CAD build for the part. Positions are in the model's coordinates, mm. Give positions to 0.01 mm unless a question says otherwise; leave off trailing zeros. Loops run counter-clockwise (first coordinate to the right, second up) from the corner with the lowest first, then second, coordinate; pieces in that order, holes last.
```python
from build123d import *

# Parameters (mm, degrees)
F_01_GASKET_DEPTH  = 1
SKETCH_2_R         = 24
F_02_HOLE_UP_DEPTH = 3
SKETCH_3_R         = 24
F_03_HOLE_LO_DEPTH = 3
SKETCH_4_R         = 4
F_04_BOLT_0_DEPTH  = 3
SKETCH_5_R         = 4
F_04_BOLT_1_DEPTH  = 3
SKETCH_6_R         = 4
F_04_BOLT_2_DEPTH  = 3
SKETCH_7_R         = 4
F_04_BOLT_3_DEPTH  = 3
SKETCH_8_R         = 4
F_04_BOLT_4_DEPTH  = 3
SKETCH_9_R         = 4
F_04_BOLT_5_DEPTH  = 3
SKETCH_10_R        = 2.5
F_05_DOWEL_0_DEPTH = 3
SKETCH_11_R        = 2.5
F_05_DOWEL_1_DEPTH = 3


with BuildPart() as part:
    # 草图1 → 01_GASKET (new body)
    with BuildSketch(Plane(origin=(-31, 0, 0), x_dir=(0, 0, -1), z_dir=(1, 0, 0))):
        with BuildLine():
            Line((-104, -40), (-62, -40))
            ThreePointArc((-62, -40), (-22, 0), (-62, 40))
            Line((-62, 40), (-104, 40))
            ThreePointArc((-104, 40), (-144, 0), (-104, -40))
        make_face()
    extrude(amount=F_01_GASKET_DEPTH)

    # 草图2 → 02_HOLE_UP (cut)
    with BuildSketch(Plane(origin=(-32, 0, 0), x_dir=(0, 0, -1), z_dir=(1, 0, 0))):
        with Locations((-104, 0)):
            Circle(SKETCH_2_R)
    extrude(amount=F_02_HOLE_UP_DEPTH, mode=Mode.SUBTRACT)

    # 草图3 → 03_HOLE_LO (cut)
    with BuildSketch(Plane(origin=(-32, 0, 0), x_dir=(0, 0, -1), z_dir=(1, 0, 0))):
        with Locations((-62, 0)):
            Circle(SKETCH_3_R)
    extrude(amount=F_03_HOLE_LO_DEPTH, mode=Mode.SUBTRACT)

    # 草图4 → 04_BOLT_0 (cut)
    with BuildSketch(Plane(origin=(-32, 0, 0), x_dir=(0, 0, -1), z_dir=(1, 0, 0))):
        with Locations((-104, 32)):
            Circle(SKETCH_4_R)
    extrude(amount=F_04_BOLT_0_DEPTH, mode=Mode.SUBTRACT)

    # 草图5 → 04_BOLT_1 (cut)
    with BuildSketch(Plane(origin=(-32, 0, 0), x_dir=(0, 0, -1), z_dir=(1, 0, 0))):
        with Locations((-104, -32)):
            Circle(SKETCH_5_R)
    extrude(amount=F_04_BOLT_1_DEPTH, mode=Mode.SUBTRACT)

    # 草图6 → 04_BOLT_2 (cut)
    with BuildSketch(Plane(origin=(-32, 0, 0), x_dir=(0, 0, -1), z_dir=(1, 0, 0))):
        with Locations((-62, 32)):
            Circle(SKETCH_6_R)
    extrude(amount=F_04_BOLT_2_DEPTH, mode=Mode.SUBTRACT)

    # 草图7 → 04_BOLT_3 (cut)
    with BuildSketch(Plane(origin=(-32, 0, 0), x_dir=(0, 0, -1), z_dir=(1, 0, 0))):
        with Locations((-62, -32)):
            Circle(SKETCH_7_R)
    extrude(amount=F_04_BOLT_3_DEPTH, mode=Mode.SUBTRACT)

    # 草图8 → 04_BOLT_4 (cut)
    with BuildSketch(Plane(origin=(-32, 0, 0), x_dir=(0, 0, -1), z_dir=(1, 0, 0))):
        with Locations((-136, 0)):
            Circle(SKETCH_8_R)
    extrude(amount=F_04_BOLT_4_DEPTH, mode=Mode.SUBTRACT)

    # 草图9 → 04_BOLT_5 (cut)
    with BuildSketch(Plane(origin=(-32, 0, 0), x_dir=(0, 0, -1), z_dir=(1, 0, 0))):
        with Locations((-30, 0)):
            Circle(SKETCH_9_R)
    extrude(amount=F_04_BOLT_5_DEPTH, mode=Mode.SUBTRACT)

    # 草图10 → 05_DOWEL_0 (cut)
    with BuildSketch(Plane(origin=(-32, 0, 0), x_dir=(0, 0, -1), z_dir=(1, 0, 0))):
        with Locations((-126.6, 22.6)):
            Circle(SKETCH_10_R)
    extrude(amount=F_05_DOWEL_0_DEPTH, mode=Mode.SUBTRACT)

    # 草图11 → 05_DOWEL_1 (cut)
    with BuildSketch(Plane(origin=(-32, 0, 0), x_dir=(0, 0, -1), z_dir=(1, 0, 0))):
        with Locations((-39.4, -22.6)):
            Circle(SKETCH_11_R)
    extrude(amount=F_05_DOWEL_1_DEPTH, mode=Mode.SUBTRACT)


solid = part.part
```
1. Saw through at A-A, the plane z = 136. List the corners of the cut face in (x, y), and give its area (3 significant figures).
Responses:
outline: (-31, -24) - (-30, -24) - (-30, -4) - (-31, -4) - close; (-31, 4) - (-30, 4) - (-30, 24) - (-31, 24) - close
area: 40.0 mm2
2. Probe line 1 along Z through (x, y) = (-30.3, 0); line 2 along Y through (x, z) = (-30.15, 104); line 3 along Z through (x, y) = (-30.45, 32). List the from-to ranges inside material, lowest first.
Responses:
line 1: z = 22 to 26, 34 to 38, 128 to 132, 140 to 144
line 2: y = -40 to -36, -28 to -24, 24 to 28, 36 to 40
line 3: z = 38 to 58, 66 to 100, 108 to 128
3. Saw through at D-D, the plane x = -30.75. Count the separate pieces of the cut face and the enclosed holes in it, and give its area (3 significant figures).
Responses:
separate pieces: 1
enclosed holes: 9
area: 4,520 mm2
4. Saw through at C-C, the plane y = 9. List the corners of the cut face in (x, z).
Responses:
outline: (-31, 23.03) - (-30, 23.03) - (-30, 39.75) - (-31, 39.75) - close; (-31, 126.25) - (-30, 126.25) - (-30, 142.97) - (-31, 142.97) - close
5. Saw through at B-B, the plane y = -32. List the corners of the cut face in (x, z).
Responses:
outline: (-31, 38) - (-30, 38) - (-30, 58) - (-31, 58) - close; (-31, 66) - (-30, 66) - (-30, 100) - (-31, 100) - close; (-31, 108) - (-30, 108) - (-30, 128) - (-31, 128) - close
6. Pull direction Y, two halves, no side cores. Call faces 1 (the face through (-30.507, -30.799, 58.185)), 2 (the face through (-31, -17, 84)), 3 (the face through (-30.51, 0.88, 143.99)): released by +Y, released by -Y, zero draft, split by the parting line, or undercut.
Responses:
face 1: undercut
face 2: zero draft
face 3: split by the parting line
